Autodesk Inventor part; units mm, degrees
ref_plane "YZ Plane" through (0, 0, 0) normal (1, 0, 0) x (0, 1, 0)
ref_plane "XZ Plane" through (0, 0, 0) normal (0, 1, 0) x (-1, 0, 0)
ref_plane "XY Plane" through (0, 0, 0) normal (0, 0, 1) x (1, 0, 0)
sketch "Sketch1" plane through (0, 0, 0) normal (0, 1, 0) x (-1, 0, 0)
  line L0 (63.5, -6.35) -> (-63.5, -6.35)
  line L1 (-63.5, -6.35) -> (-63.5, 6.35)
  line L2 (-63.5, 6.35) -> (63.5, 6.35)
  line L3 (63.5, 6.35) -> (63.5, -6.35)
  line L4 (63.5, -6.35) -> (-63.5, 6.35) construction
  line L5 (-63.5, -6.35) -> (63.5, 6.35) construction
  point P0 (0, 0)
  dimension "d0" = 12.7
  dimension "d1" = 127
extrude "Extrusion1" add sketch "Sketch1" along normal blind 22.225
sketch "Sketch2" plane through (-63.5, 0, 6.35) normal (0, 0, 1) x (1, 0, 0)
  line L0 (127, 0) -> (0, 0)
  line L1 (127, 0) -> (127, 22.225)
  line L2 (0, 22.225) -> (127, 22.225)
  line L3 (0, 0) -> (0, 22.225)
  line L4 (6.35, 22.225) -> (120.65, 22.225)
  line L5 (120.65, 22.225) -> (120.65, 9.525)
  line L6 (120.65, 9.525) -> (6.35, 9.525)
  line L7 (6.35, 9.525) -> (6.35, 22.225)
  point P0 (63.5, 0)
  dimension "d4" = 6.35
  dimension "d5" = 6.35
  dimension "d6" = 9.525
extrude "Extrusion2" cut sketch "Sketch2" against normal blind 22.225 contours L5 L6 L7 L2
fillet "Fillet1" radius 6.35 2 edges at (57.15, 9.525, 0) (-57.15, 9.525, 0)
sketch "Sketch3" plane through (-57.15, 22.225, 6.35) normal (1, 0, 0) x (0, 0, -1)
  line L0 (0, 0) -> (12.7, 0)
  point P0 (6.35, -22.225)
  point P1 (6.35, -8.255)
  dimension "d10" = 8.255
hole "Hole1" at (-57.15, 13.97, 0) direction (-1, 0, 0) diameter 3.683 end through all
sketch "Sketch4" plane through (-63.5, 0, -6.35) normal (-1, 0, 0) x (0, 0, 1)
  circle A0 centre (6.35, 13.97) radius 1.8415
  point P0 (6.35, 0)
hole "Hole2" at (-63.5, 13.97, 0) direction (1, 0, 0) diameter 3.683 end through all
sketch "Sketch5" plane through (57.15, 22.225, -6.35) normal (-1, 0, 0) x (0, 0, 1)
  circle A0 centre (6.35, -8.255) radius 1.8415
  circle A1 centre (6.35, -8.255) radius 4.064
  point P0 (6.35, -22.225)
  dimension "d25" = 8.128
extrude "Extrusion3" cut sketch "Sketch5" along normal blind 22.225
fillet "Fillet2" radius 3.175 4 edges at (60.325, 22.225, 6.35) (60.325, 22.225, -6.35) (-60.325, 22.225, 6.35) (-60.325, 22.225, -6.35)
sketch "Sketch6" plane through (-57.15, 15.875, 6.35) normal (1, 0, 0) x (0, 0, -1)
  circle A0 centre (6.35, -1.905) radius 1.8415
  circle A1 centre (6.35, -1.905) radius 4.064
  point P0 (6.35, -15.875)
  dimension "d29" = 8.128
extrude "Extrusion4" cut sketch "Sketch6" along normal blind 22.225
fillet "Fillet3" radius 1.27 16 edges at (-55.2901, 11.3849, 6.35) (-57.15, 17.4625, 6.35) (-57.15, 21.2951, 5.4201) (-57.15, 22.225, 0) (-57.15, 21.2951, -5.4201) (-57.15, 17.4625, -6.35) (-55.2901, 11.3849, -6.35) (0, 9.525, -6.35) (55.2901, 11.3849, -6.35) (57.15, 17.4625, -6.35) (57.15, 21.2951, -5.4201) (57.15, 22.225, 0) (57.15, 21.2951, 5.4201) (57.15, 17.4625, 6.35) (55.2901, 11.3849, 6.35) (0, 9.525, 6.35)
properties part number "SwarmieLidSupport"
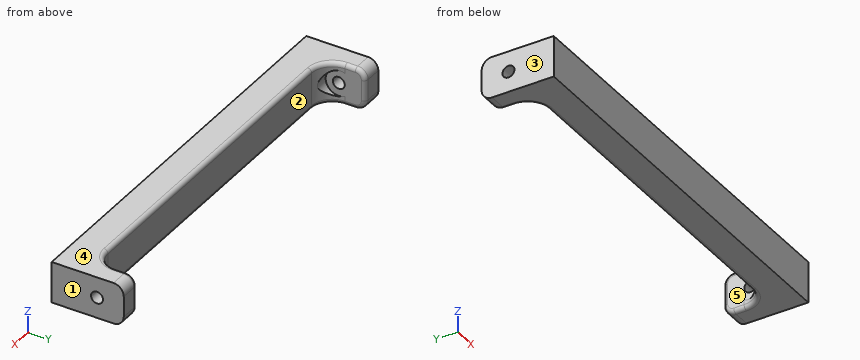
CAD build for the part. Positions are in the model's coordinates, mm. Face numbers are marked on the shaded views. A direction names the side the tool comes from. Round coordinates to 2 decimals unless told otherwise and drop trailing zeros. Loops run counter-clockwise (first coordinate to the right, second up) from the corner with the lowest first, then second, coordinate; pieces in that order, holes last. Notation, with made-up numbers: (59, 69) - (109, 69) arc R27 ccw to (109, 105) - close; hole circle Ø5 at (-5.5, 19.25). An arc over 180 degrees is marked (long way). Put each result on its own line as item: value.
1. Two-plate mould, pull along X, no slides. Class the marked faces 3, 4 and 5: released by +X, released by -X, zero draft, split by the parting line, or undercut.
Geometry check:
face 3: released by -X
face 4: zero draft
face 5: undercut
2. Wall check: line 1 (X direction, y = 11.5, z = 0.75); line 2 (Y direction, x = 61.5, z = 0) (1 decimal); line 3 (Y direction, x = -8, z = 4.25) (3 decimals). Give the ranges that are in metal, low to high.
Geometry check:
line 1: -63.5 to -57.15, 57.15 to 63.5
line 2: 0 to 12.1, 15.8 to 22.2
line 3: 0 to 9.525
3. Slice it at B-B on z = 0. Give the number of separate pieces and of enclosed holes in the cut face, and give its area (3 significant figures).
Geometry check:
separate pieces: 3
enclosed holes: 0
area: 1,330 mm²
4. Slice it at C-C on x = -18. List the corners of the cut face in (y, z) (3 decimals), and give its area (3 significant figures).
Geometry check:
outline: (0, -6.35) - (8.255, -6.35) arc R1.27 ccw to (9.525, -5.08) - (9.525, 5.08) arc R1.27 ccw to (8.255, 6.35) - (0, 6.35) - close
area: 120 mm²
5. Pin check, flat tips, straight feed: P1, Ø5, axis at y = 13.97, z = 0, coming from the +X side; P2, Ø3, axis at x = -4, z = -1.5, coming from the +Y side (3 decimals). Stop position of each tip, or through.
Geometry check:
P1: x = 63.5
P2: y = 9.525
6. Slice it at A-A on y = 17. List the corners of the cut face in (x, z), and give its area (3 significant figures).
Geometry check:
outline: (-63.5, -6.35) - (-58.42, -6.35) arc R1.27 ccw to (-57.15, -5.08) - (-57.15, 5.08) arc R1.27 ccw to (-58.42, 6.35) - (-63.5, 6.35) - close; (57.15, -5.08) arc R1.27 ccw to (58.42, -6.35) - (63.5, -6.35) - (63.5, 6.35) - (58.42, 6.35) arc R1.27 ccw to (57.15, 5.08) - close
area: 160 mm²
7. 3-axis set-ups, long thin cutter, end or side, ignore diameter. For the marked faces 1 and 2: which of +Z, -Z, +X, -X, +Y, -Y reach the whole face in a straight line?
Geometry check:
face 1: +Z, -Z, +X, +Y, -Y
face 2: +Z, -Z, +Y
